Geometry: see drawing. Coordinates: mm, zero at the bounding-box minimum. Give positions to 0.01 mm unless a question says otherwise; leave off trailing zeros. Write each loop counter-clockwise with the first axis right and the second up, starting at its lowest first coordinate (ties: lowest second). Pieces come first, ordered by that corner, then holes. Notation, with made-up numbers: M 51,27.25 L 99,27.25 A30 cw 99,59.25 Z; hole C 41,28 d2. An arc over 180 degrees is marked long. Use CSV: the item, a comma, the result in double quotes. Start each with the question number.
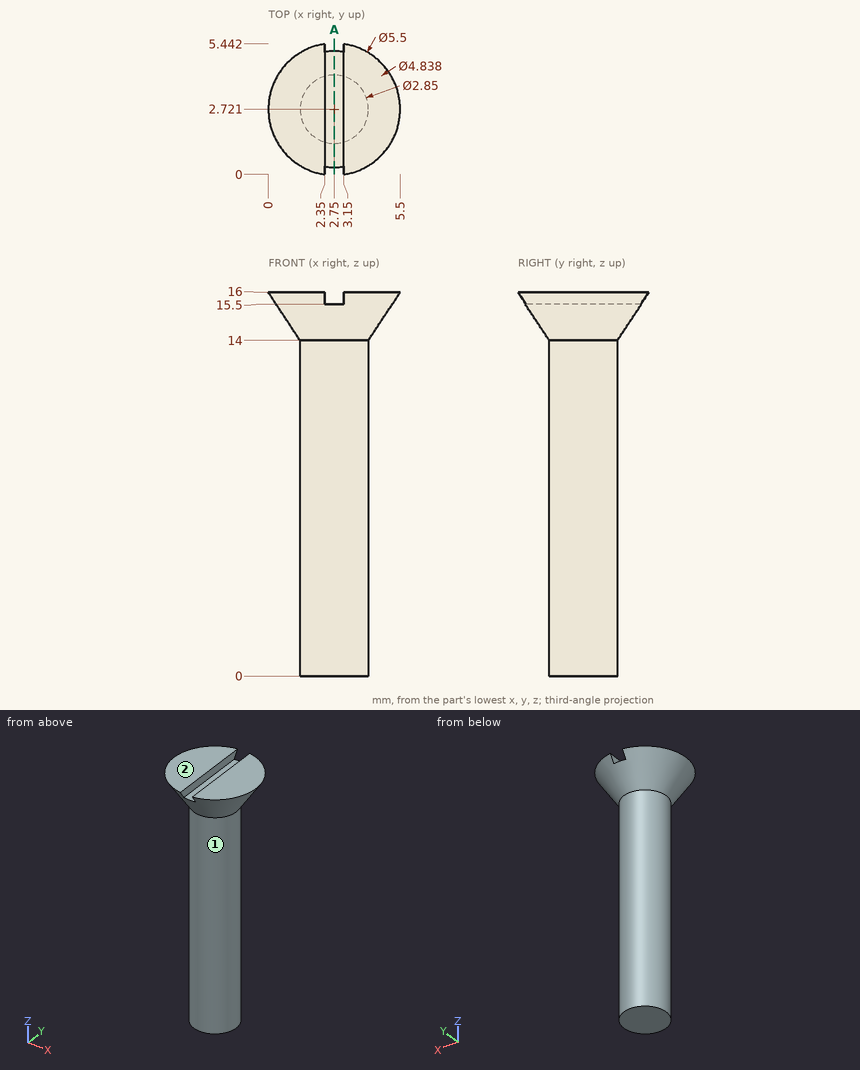
1. First-contact query: pin 1 (2 mm diameter, centred on y = 1, z = 4.5, fed in from +X); pin 2 (1 mm diameter, centred on x = 4.5, y = 4.5, fed in from -Z); pin 3 (1 mm diameter, centred on y = 3.5, z = 8, fed in from -X); pin 4 (1.5 mm diameter, centred on x = 3, y = 2, fed in from +Z). Flat tips, straight axial feed; report the tip coordinate or a pass-through.
2. Section A-A on x = 2.75. Return loops of the section in (y, z) (1 decimal).
3. Pull-direction query (X, two-part tool) for the marked faces 1 and 2; classes: released by +X, released by -X, zero draft, split by the parting line, or undercut.
4. Line query: probe 1 along Z at (x, y) = (2.65, 3.05); probe 2 along X at (y, z) = (2.8, 4); probe 3 along X at (y, z) = (3.1, 11.25) (1 decimal). Output: solid intervals per line, ascending.
Resolved:
1,pin 1,"stops at x = 3.98"
1,pin 2,"stops at z = 14.86"
1,pin 3,"stops at x = 1.35"
1,pin 4,"stops at z = 16"
2,outline,"M 0.3,15.5 L 1.3,14 L 1.3,0 L 4.1,0 L 4.1,14 L 5.1,15.5 Z"
3,face 1,"split by the parting line"
3,face 2,"zero draft"
4,probe 1,"z = 0 to 15.5"
4,probe 2,"x = 1.33 to 4.17"
4,probe 3,"x = 1.4 to 4.1"
